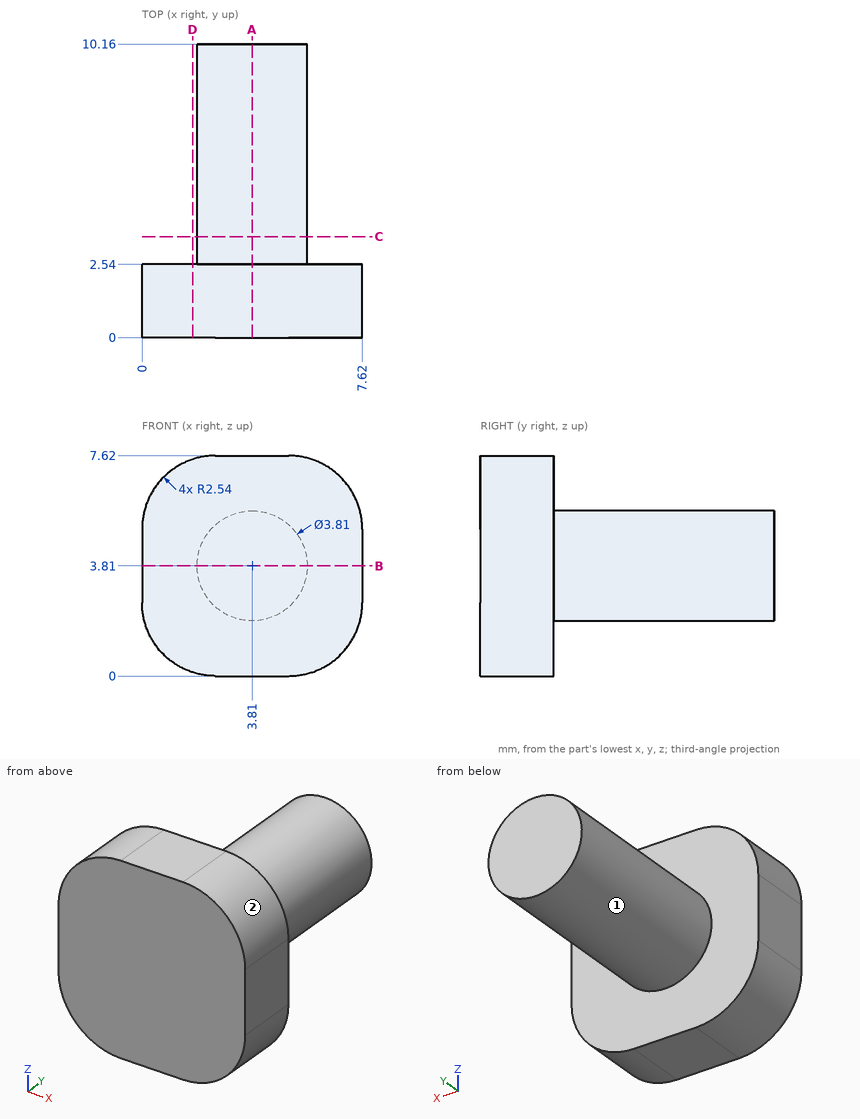
Answer from the drawing. Dimensions are ordinates in mm from the lowest x, y and z of the part. A direction names the side the tool comes from. Give positions to 0.01 mm unless a question says otherwise; leave off trailing zeros. Write each loop counter-clockwise with the first axis right and the second up, starting at its lowest first coordinate (ties: lowest second). Pieces come first, ordered by that corner, then holes. Notation, with made-up numbers: (35.25, 62) - (92.25, 62) arc R25 ccw to (92.25, 97) - close; hole circle Ø7 at (27, -32.75). An arc over 180 degrees is marked (long way). One line per item, written item: value. Start each with the question number.
1. Consider probe 1 along Y at (x, z) = (1.5, 7); probe 2 along Z at (x, y) = (0.5, 2); probe 3 along X at (y, z) = (4.5, 5). Determine where each line is inside the solid, lowest interval first.
2. For the marked faces 1 and 2, determine the directions among +Z, -Z, +X, -X, +Y, -Y from which every point of the face is accessible in a straight line to the end or side of a thin tool.
3. Find section B-B (z = 3.81). Write down the section's boundary in (x, y) (3 decimals).
4. Find section A-A (x = 3.81). Write down the section's boundary in (y, z) (3 decimals), then the cut area to 3 significant figures.
5. Given pin 1 (1 mm diameter, centred on x = 6.5, z = 3, fed in from +Y); pin 2 (2 mm diameter, centred on x = 2, y = 7.5, fed in from +Z), each flat-ended and moving along its own axis, determine where each tip first touches the part or whether it passes through.
6. Find section D-D (x = 1.75). Write down the section's boundary in (y, z), then the cut area to 3 significant figures.
7. Find section C-C (y = 3.5). Write down the section's boundary in (x, z) (3 decimals), then the cut area to 3 significant figures.
Geometry results:
1. probe 1: 0 to 2.54
1. probe 2: 1.03 to 6.59
1. probe 3: 2.32 to 5.3
2. face 1: +Y
2. face 2: +Z, +X, +Y, -Y
3. outline: (0, 0) - (7.62, 0) - (7.62, 2.54) - (5.715, 2.54) - (5.715, 10.16) - (1.905, 10.16) - (1.905, 2.54) - (0, 2.54) - close
4. outline: (0, 0) - (2.54, 0) - (2.54, 1.905) - (10.16, 1.905) - (10.16, 5.715) - (2.54, 5.715) - (2.54, 7.62) - (0, 7.62) - close
4. area: 48.4 mm2
5. pin 1: y = 2.54
5. pin 2: z = 5.53
6. outline: (0, 0.13) - (2.54, 0.13) - (2.54, 7.49) - (0, 7.49) - close
6. area: 18.7 mm2
7. outline: circle Ø3.81 at (3.81, 3.81)
7. area: 11.4 mm2
